```python
from build123d import *

# Parameters (mm, degrees)
BOSS_EXTRUDE1_DEPTH = 2
SKETCH2_R           = 7.625
BOSS_EXTRUDE2_DEPTH = 14
SKETCH3_R           = 6.604
BOSS_EXTRUDE3_DEPTH = 4
BOSS_EXTRUDE4_START = 3.175
BOSS_EXTRUDE4_DEPTH = 3


with BuildPart() as part:
    # Sketch1 → Boss-Extrude1 (new body)
    with BuildSketch(Plane(origin=(0, 0, 0), x_dir=(0, 0, -1), z_dir=(1, 0, 0))):
        Polygon((5.196152442, 9.000000034), (-5.196152442, 9.000000034), (-10.392304885, 0), (-5.196152442, -9.000000034), (5.196152442, -9.000000034), (10.392304885, 0), align=None)
    extrude(amount=BOSS_EXTRUDE1_DEPTH)

    # Sketch2 → Boss-Extrude2 (add)
    with BuildSketch(Plane(origin=(2, 0, 0), x_dir=(0, 0, -1), z_dir=(1, 0, 0))):
        Circle(SKETCH2_R)
    extrude(amount=BOSS_EXTRUDE2_DEPTH)

    # Sketch3 → Boss-Extrude3 (add)
    with BuildSketch(Plane(origin=(16, 0, 0), x_dir=(0, 0, -1), z_dir=(1, 0, 0))):
        Circle(SKETCH3_R)
    extrude(amount=BOSS_EXTRUDE3_DEPTH)

    # Sketch4 → Boss-Extrude4 (add)
    with BuildSketch(Plane(origin=(2, 0, 0), x_dir=(0, 0, -1), z_dir=(1, 0, 0)).offset(BOSS_EXTRUDE4_START)):
        Polygon((10.392304885, 0), (5.196152442, 9.000000034), (-5.196152442, 9.000000034), (-10.392304885, 0), (-5.196152442, -9.000000034), (5.196152442, -9.000000034), align=None)
    extrude(amount=BOSS_EXTRUDE4_DEPTH)


solid = part.part
```
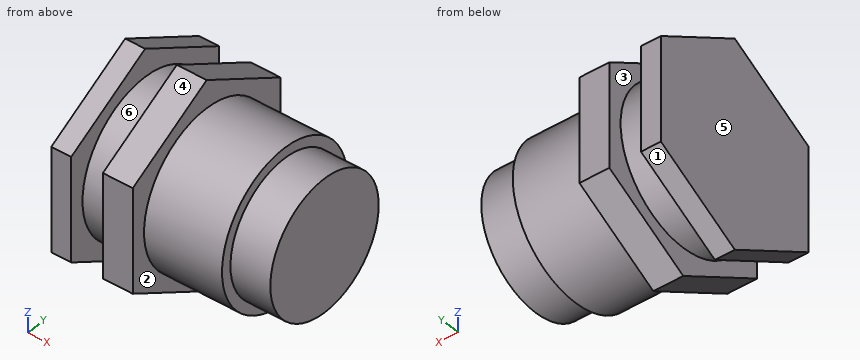
Could you check a few things on this model? Use its own coordinates, in mm. Face numbers are marked on the shaded views. A direction names the side the tool comes from. Give positions to 0.01 mm unless a question says otherwise; leave off trailing zeros. Write each loop counter-clockwise with the first axis right and the second up, starting at its lowest first coordinate (ties: lowest second). Pieces come first, ordered by that corner, then holes. Notation, with made-up numbers: (52, 26.5) - (59, 26.5) arc R15 cw to (59, 35.5) - close; hole circle Ø2 at (1, 1). An arc over 180 degrees is marked (long way). One line per item, written item: value. Start each with the question number.
Item 1: Please list where these lines run through material, in increasing order: line 1 (X direction, y = -3.75, z = 7.75) (3 decimals); line 2 (X direction, y = 7.25, z = -1.25); line 3 (Y direction, x = 3, z = 0) (3 decimals). Write a range as from..to.
Item 2: Imagine slicing it at D-D, the plane y = 0.5. List the corners of the cut face in (x, z) for me (3 decimals).
Item 3: If we mould it in two halves opening along X, with no side actions, what happens to the marked faces 4, 5 and 6? For each: +X half, -X half, draft (parallel to the pull), parting line (faces both ways), or undercut.
Item 4: Imagine slicing it at A-A, the plane x = 6.75. List the corners of the cut face in (y, z) for me.
Item 5: I'm going to push flat-ended pins straight in: pin 1 (5 mm diameter, centred on x = 11.5, z = -6.5, fed in from +Y); pin 2 (6 mm diameter, centred on x = 13, z = 2.5, fed in from +Y) (3 decimals); pin 3 (10 mm diameter, centred on x = 16.5, y = 7, fed in from -Z). Where does each tip first touch, or does it pass through?
Item 6: Imagine slicing it at C-C, the plane z = -2.5. List the corners of the cut face in (x, y) for me (3 decimals), and give its area (3 significant figures).
Item 7: Imagine slicing it at B-B, the plane y = -8. List the corners of the cut face in (x, z) for me (1 decimal), and give its area (3 significant figures).
Item 8: Which directions (+Z, -Z, +X, -X, +Y, -Y) give clear straight access to the entire face, cutting with the end or side of a thin tool? Please do the marked faces 1, 2 and 3.
Geometry says:
1. line 1: 0..2, 5.175..8.175
1. line 2: 0..16
1. line 3: -7.625..7.625
2. outline: (0, -10.104) - (2, -10.104) - (2, -7.609) - (5.175, -7.609) - (5.175, -10.104) - (8.175, -10.104) - (8.175, -7.609) - (16, -7.609) - (16, -6.585) - (20, -6.585) - (20, 6.585) - (16, 6.585) - (16, 7.609) - (8.175, 7.609) - (8.175, 10.104) - (5.175, 10.104) - (5.175, 7.609) - (2, 7.609) - (2, 10.104) - (0, 10.104) - close
3. face 4: draft
3. face 5: -X half
3. face 6: undercut
4. outline: (-9, -5.2) - (0, -10.39) - (9, -5.2) - (9, 5.2) - (0, 10.39) - (-9, 5.2) - close
5. pin 1: y = 6.49
5. pin 2: y = 7.625
5. pin 3: z = -7.35
6. outline: (0, -9) - (2, -9) - (2, -7.204) - (5.175, -7.204) - (5.175, -9) - (8.175, -9) - (8.175, -7.204) - (16, -7.204) - (16, -6.113) - (20, -6.113) - (20, 6.113) - (16, 6.113) - (16, 7.204) - (8.175, 7.204) - (8.175, 9) - (5.175, 9) - (5.175, 7.204) - (2, 7.204) - (2, 9) - (0, 9) - close
6. area: 297 mm^2
7. outline: (0, -5.8) - (2, -5.8) - (2, 5.8) - (0, 5.8) - close; (5.2, -5.8) - (8.2, -5.8) - (8.2, 5.8) - (5.2, 5.8) - close
7. area: 57.7 mm^2
8. face 1: -Z, +X, -X, +Y
8. face 2: +X
8. face 3: none
